For this review, use the dimensioned drawing (mm, ordinates from the lowest corner) and the shaded views. A direction names the side the tool comes from. Round coordinates to 2 decimals unless told otherwise and drop trailing zeros. Write each loop counter-clockwise with the first axis right and the second up, starting at its lowest first coordinate (ties: lowest second). Pieces come first, ordered by that corner, then holes. Notation, with made-up numbers: M 9,76 L 48,76 A25 ccw 48,111 Z; hole C -17,87 d2. An arc over 180 degrees is marked long. One line per question, with ' | ' between items. Start each with the question number.
Item 1: Add section C-C, the plane x = 30. State the section outline as (y, z) points.
Item 2: For L1, parallel to X at y = 2.25, z = 10; L2, parallel to X at y = 1.05, z = 10; L3, parallel to Z at x = 30, y = 1.9, list the stretches that pass through material, from the lowest coordinate up.
Item 3: Insertion check: pin 1 Ø6 at (x, z) = (30, 10) entering from -Y; pin 2 Ø5 at (y, z) = (9.5, 4.5) entering from -X; pin 3 Ø2.5 at (x, y) = (21, 9) entering from -Z. Each pin has a flat end and moves straight along its axis. Give the tip position at first contact, or say it passes through.
Item 4: Add section A-A, the plane y = 1. State the section outline as (x, z) points, and give its area (3 significant figures).
Item 5: Machinability: for the marked faces 1, 2, 3, 4 and 5, which of the approach directions +Z, -Z, +X, -X, +Y, -Y give a long, thin tool a straight path to every point of the face, cutting with its end or side? Answer none if there is none.
Item 6: Add section B-B, the plane z = 10. State the section outline as (x, y) points.
Item 7: Add section D-D, the plane y = 4.25. State the section outline as (x, z) points.
Item 8: Draft analysis for pull direction X (two halves, no side actions). For the marked faces 6, 7 and 8, state which applies: released by +X, released by -X, zero draft, split by the parting line, or undercut.
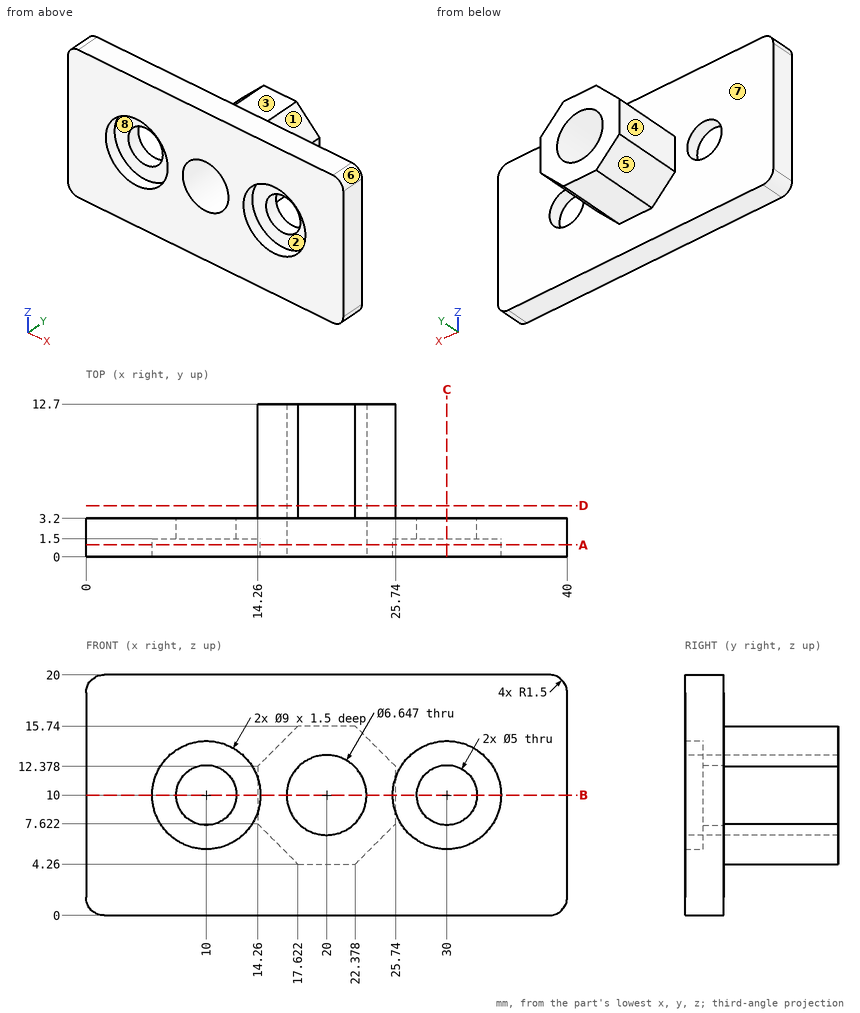
Computed values:
1) outline: M 0,0 L 3.2,0 L 3.2,7.5 L 1.5,7.5 L 1.5,5.5 L 0,5.5 Z; M 0,14.5 L 1.5,14.5 L 1.5,12.5 L 3.2,12.5 L 3.2,20 L 0,20 Z
2) L1: x = 0 to 7.5, 12.5 to 16.68, 23.32 to 27.5, 32.5 to 40 | L2: x = 0 to 5.5, 14.5 to 16.68, 23.32 to 25.5, 34.5 to 40 | L3: z = 0 to 7.5, 12.5 to 20
3) pin 1: stops at y = 1.5 | pin 2: stops at x = 14.88 | pin 3: stops at z = 4.26
4) outline: M 0,1.5 A1.5 ccw 1.5,0 L 38.5,0 A1.5 ccw 40,1.5 L 40,18.5 A1.5 ccw 38.5,20 L 1.5,20 A1.5 ccw 0,18.5 Z; hole C 10,10 d9; hole C 20,10 d6.65; hole C 30,10 d9 | area: 636 mm^2
5) face 1: +Z, +X, +Y | face 2: -Y | face 3: +Z, +X, -X, +Y | face 4: +Z, -Z, -X, +Y | face 5: -Z, -X, +Y
6) outline: M 0,0 L 5.5,0 L 5.5,1.5 L 7.5,1.5 L 7.5,3.2 L 0,3.2 Z; M 12.5,1.5 L 14.5,1.5 L 14.5,0 L 16.68,0 L 16.68,12.7 L 14.26,12.7 L 14.26,3.2 L 12.5,3.2 Z; M 23.32,0 L 25.5,0 L 25.5,1.5 L 27.5,1.5 L 27.5,3.2 L 25.74,3.2 L 25.74,12.7 L 23.32,12.7 Z; M 32.5,1.5 L 34.5,1.5 L 34.5,0 L 40,0 L 40,3.2 L 32.5,3.2 Z
7) outline: M 14.26,7.62 L 17.62,4.26 L 22.38,4.26 L 25.74,7.62 L 25.74,12.38 L 22.38,15.74 L 17.62,15.74 L 14.26,12.38 Z; hole C 20,10 d6.65
8) face 6: released by +X | face 7: zero draft | face 8: undercut
